CAD build for the part. Positions are in the model's coordinates, mm. Face numbers are marked on the shaded views. A direction names the side the tool comes from. Round coordinates to 2 decimals unless told otherwise and drop trailing zeros. Loops run counter-clockwise (first coordinate to the right, second up) from the corner with the lowest first, then second, coordinate; pieces in that order, holes last. Notation, with made-up numbers: M 18.25,-6 L 72.25,-6 A25 cw 72.25,7 Z; hole C -10,34.25 d1. An arc over 180 degrees is marked long. Use a Markdown table: item, result. Add a question column.
(1) Band-saw the part on D-D, the plane y = -20.5. Write the cut outline in (x, z) (3 decimals), and give its area (3 significant figures).
(2) Band-saw the part on C-C, the plane z = 0.75. Give the number of separate pieces and of enclosed holes in the cut face, and give its area (3 significant figures).
(3) Two-plate mould, pull along Y, no slides. Class the marked faces 3, 4 and 5: released by +Y, released by -Y, zero draft, split by the parting line, or undercut.
(4) Flat gauge pins, fed straight in: P1, Ø5, axis at x = 22.5, y = 15, coming from the +Z side (3 decimals); P2, Ø1, axis at x = 34.5, z = 6, coming from the +Y side; P3, Ø5, axis at y = -22.5, z = 3.5, coming from the +X side; P4, Ø3, axis at y = -39, z = 2, coming from the -X side. Where does each tip first touch, or does it go through?
(5) Band-saw the part on A-A, the plane x = 25.4. Write the cut outline in (y, z) (3 decimals).
(6) Which spindle directions (+Z, -Z, +X, -X, +Y, -Y) get a long thin tool onto all of the face, cutting with end or side? Do the marked faces 1 and 2. Say none if no direction does.
(7) Wall check: L1, parallel to Y at x = 25.4, z = 5.5; L2, parallel to X at y = -38.1, z = 6.25; L3, parallel to X at y = -28.5, z = 6.5. Give the ranges that are in metal, low to high.
(8) Band-saw the part on B-B, the plane y = 12.7. Write the cut outline in (x, z) (3 decimals).
from build123d import *

# Parameters (mm, degrees)
SKETCH1_R           = 6.35
BOSS_EXTRUDE1_DEPTH = 9.525
SKETCH2_R           = 6.35
CUT_EXTRUDE1_DEPTH  = 73.470722537
FILLET1_R           = 12.7
FILLET2_R           = 1


with BuildPart() as part:
    # Sketch1 → Boss-Extrude1 (new body)
    with BuildSketch(Plane.XY):
        with BuildLine():
            Line((0, 0), (12.7, 0))
            Line((12.7, 0), (12.7, -38.1))
            ThreePointArc((12.7, -38.1), (25.4, -50.8), (38.1, -38.1))
            Line((38.1, -38.1), (38.1, 0))
            Line((38.1, 0), (50.8, 0))
            ThreePointArc((50.8, 0), (25.4, 25.4), (0, 0))
        make_face()
        with Locations(Location((25.4, -38.1, 0), (0, 0, 180))):
            Circle(SKETCH1_R, mode=Mode.SUBTRACT)
    extrude(amount=BOSS_EXTRUDE1_DEPTH)

    # Sketch2 → Cut-Extrude1 (cut, through all)
    with BuildSketch(Plane.XY.offset(9.525)):
        with Locations((25.4, 12.7)):
            Circle(SKETCH2_R)
    extrude(amount=-CUT_EXTRUDE1_DEPTH, mode=Mode.SUBTRACT)

    # Fillet1
    fillet1_edges = [part.edges().sort_by_distance(p)[0] for p in [
        (38.1, 0, 4.7625),
        (12.7, 0, 4.7625),
    ]]
    fillet(fillet1_edges, radius=FILLET1_R - 0.0001)  # a hair under: the kernel refuses the full size

    # Fillet2
    fillet2_edges = [part.edges().sort_by_distance(p)[0] for p in [
        (0, 0, 4.7625),
        (50.8, 0, 4.7625),
    ]]
    fillet(fillet2_edges, radius=FILLET2_R)


solid = part.part
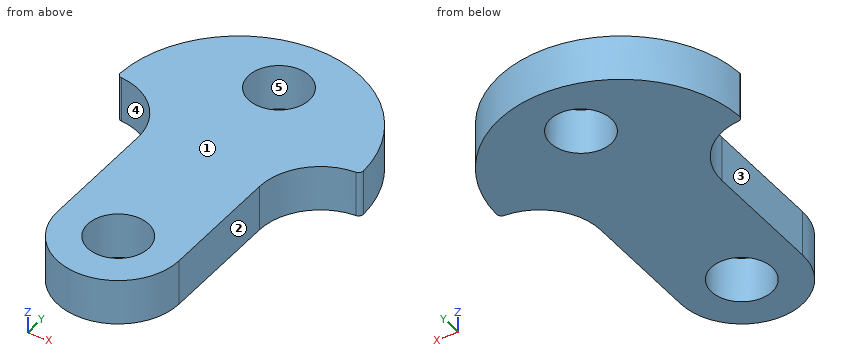
Return value:
| question | item | result |
|---|---|---|
| 1 | outline | M 12.7,0 L 38.1,0 L 38.1,9.525 L 12.7,9.525 Z |
| 1 | area | 242 mm^2 |
| 2 | separate pieces | 1 |
| 2 | enclosed holes | 2 |
| 2 | area | 2,050 mm^2 |
| 3 | face 3 | zero draft |
| 3 | face 4 | released by -Y |
| 3 | face 5 | undercut |
| 4 | P1 | through |
| 4 | P2 | y = 23.9 |
| 4 | P3 | x = 38.1 |
| 4 | P4 | x = 12.7 |
| 5 | outline | M -50.8,0 L -44.45,0 L -44.45,9.525 L -50.8,9.525 Z; M -31.75,0 L 6.35,0 L 6.35,9.525 L -31.75,9.525 Z; M 19.05,0 L 25.4,0 L 25.4,9.525 L 19.05,9.525 Z |
| 6 | face 1 | +Z, +X, -X, +Y, -Y |
| 6 | face 2 | +Z, -Z, +X, -Y |
| 7 | L1 | -50.8 to -44.45, -31.75 to 6.35, 19.05 to 25.4 |
| 7 | L2 | 12.7 to 19.05, 31.75 to 38.1 |
| 7 | L3 | 12.7 to 38.1 |
| 8 | outline | M 3.403,0 L 19.05,0 L 19.05,9.525 L 3.403,9.525 Z; M 31.75,0 L 47.397,0 L 47.397,9.525 L 31.75,9.525 Z |
